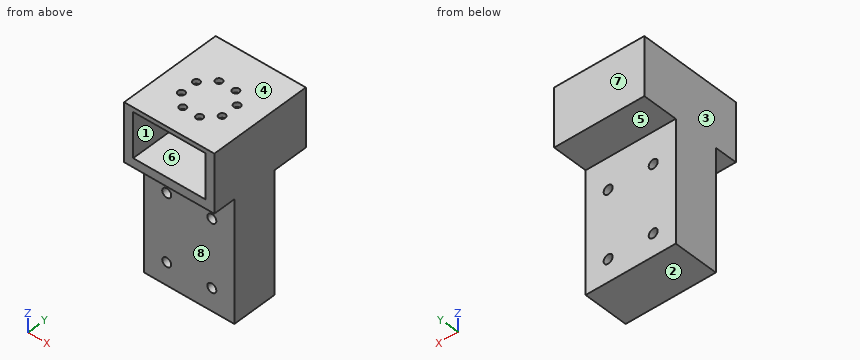
from build123d import *

# Parameters (mm, degrees)
CROQUIS1_W              = 40
CROQUIS1_H              = 40
SALIENTE_EXTRUIR1_DEPTH = 4
CROQUIS2_R              = 1.5
CORTAR_EXTRUIR1_DEPTH   = 4
SALIENTE_EXTRUIR2_DEPTH = 20
CROQUIS4_W              = 40
CROQUIS4_H              = 40
SALIENTE_EXTRUIR3_DEPTH = 4
CROQUIS6_W              = 40
CROQUIS6_H              = 40
CORTAR_EXTRUIR3_DEPTH   = 2
CROQUIS7_W              = 40
CROQUIS7_H              = 20
SALIENTE_EXTRUIR4_DEPTH = 80
CROQUIS8_R              = 2
CORTAR_EXTRUIR4_DEPTH   = 31
CROQUIS9_R              = 2
CORTAR_EXTRUIR5_DEPTH   = 31
CROQUIS11_W             = 40
CROQUIS11_H             = 20
CORTAR_EXTRUIR6_DEPTH   = 26
CROQUIS13_W             = 40
CROQUIS13_H             = 26
SALIENTE_EXTRUIR5_DEPTH = 5.7


with BuildPart() as part:
    # Croquis1 → Saliente-Extruir1 (new body)
    with BuildSketch(Plane.XY):
        Rectangle(CROQUIS1_W, CROQUIS1_H)
    extrude(amount=SALIENTE_EXTRUIR1_DEPTH)

    # Croquis2 → Cortar-Extruir1 (cut)
    with BuildSketch(Plane.XY.offset(4)):
        with Locations((-9.034617948, -3.742261285)):
            Circle(CROQUIS2_R)
        with Locations((-9.034617948, 3.742261285)):
            Circle(CROQUIS2_R)
        with Locations((-3.742261285, 9.034617948)):
            Circle(CROQUIS2_R)
        with Locations((3.742261285, 9.034617948)):
            Circle(CROQUIS2_R)
        with Locations((9.034617948, 3.742261285)):
            Circle(CROQUIS2_R)
        with Locations((9.034617948, -3.742261285)):
            Circle(CROQUIS2_R)
        with Locations((3.742261285, -9.034617948)):
            Circle(CROQUIS2_R)
        with Locations((-3.742261285, -9.034617948)):
            Circle(CROQUIS2_R)
    extrude(amount=-CORTAR_EXTRUIR1_DEPTH, mode=Mode.SUBTRACT)

    # Croquis3 → Saliente-Extruir2 (add)
    with BuildSketch(Plane(origin=(0, 0, 0), x_dir=(-1, 0, 0), z_dir=(0, 0, -1))):
        Polygon((-16, -20), (-16, -16), (-16, 16), (16, 16), (16, -16), (16, -20), (20, -20), (20, 20), (-20, 20), (-20, -20), align=None)
    extrude(amount=SALIENTE_EXTRUIR2_DEPTH)

    # Croquis4 → Saliente-Extruir3 (add)
    with BuildSketch(Plane(origin=(0, 0, -20), x_dir=(-1, 0, 0), z_dir=(0, 0, -1))):
        Rectangle(CROQUIS4_W, CROQUIS4_H)
    extrude(amount=SALIENTE_EXTRUIR3_DEPTH)

    # Croquis6 → Cortar-Extruir3 (cut)
    with BuildSketch(Plane.XY.offset(4)):
        Rectangle(CROQUIS6_W, CROQUIS6_H)
    extrude(amount=-CORTAR_EXTRUIR3_DEPTH, mode=Mode.SUBTRACT)

    # Croquis7 → Saliente-Extruir4 (add)
    with BuildSketch(Plane(origin=(0, 0, -24), x_dir=(-1, 0, 0), z_dir=(0, 0, -1))):
        Rectangle(CROQUIS7_W, CROQUIS7_H)
    extrude(amount=SALIENTE_EXTRUIR4_DEPTH)

    # Croquis8 → Cortar-Extruir4 (cut, through all)
    with BuildSketch(Plane(origin=(0, 10, 0), x_dir=(1, 0, 0), z_dir=(0, 1, 0))):
        with Locations((-10, 38)):
            Circle(CROQUIS8_R)
        with Locations((10, 38)):
            Circle(CROQUIS8_R)
    extrude(amount=-CORTAR_EXTRUIR4_DEPTH, mode=Mode.SUBTRACT)

    # Croquis9 → Cortar-Extruir5 (cut, through all)
    with BuildSketch(Plane(origin=(0, 10, 0), x_dir=(1, 0, 0), z_dir=(0, 1, 0))):
        with Locations((10, 68)):
            Circle(CROQUIS9_R)
        with Locations((-10, 68)):
            Circle(CROQUIS9_R)
    extrude(amount=-CORTAR_EXTRUIR5_DEPTH, mode=Mode.SUBTRACT)

    # Croquis11 → Cortar-Extruir6 (cut)
    with BuildSketch(Plane(origin=(0, 0, -104), x_dir=(-1, 0, 0), z_dir=(0, 0, -1))):
        Rectangle(CROQUIS11_W, CROQUIS11_H)
    extrude(amount=-CORTAR_EXTRUIR6_DEPTH, mode=Mode.SUBTRACT)

    # Croquis13 → Saliente-Extruir5 (add)
    with BuildSketch(Plane(origin=(0, 20, 0), x_dir=(1, 0, 0), z_dir=(0, 1, 0))):
        with Locations((0, 11)):
            Rectangle(CROQUIS13_W, CROQUIS13_H)
    extrude(amount=SALIENTE_EXTRUIR5_DEPTH)


solid = part.part
Geometry check sheet. Reference: the model listing, model coordinates, mm. Face numbers are marked on the shaded views. A direction names the side the tool comes from. Coordinates: 2 decimals unless noted, no trailing zeros. Loops run counter-clockwise (first coordinate to the right, second up) from the corner with the lowest first, then second, coordinate; pieces in that order, holes last. Notation, with made-up numbers: (-26, -39) - (10, -39) arc R20 ccw to (10, -9) - close; hole circle Ø5 at (78, 39.25). An arc over 180 degrees is marked (long way). Use one line per item in the form item = value. Start each with the question number.
Item 1: Thickness scan on probe 1 along Z at (x, y) = (10, 5); probe 2 along X at (y, z) = (4.75, -38); probe 3 along Z at (x, y) = (-5, -7.5). Record the ranges inside material, lowest first.
Item 2: Section check A-A, the plane z = -68. Enter the section's corners in (x, y).
Item 3: Mould release check, pull along Z, two halves, no side actions. Record for the marked faces 1, 2, 3 and 4: +Z half, -Z half, draft (parallel to the pull), parting line (faces both ways), or undercut.
Item 4: Section check B-B, the plane x = 17. Enter the section's corners in (y, z).
Item 5: Tool access check on the marked faces 5, 6, 7 and 8. Record the directions out of +Z, -Z, +X, -X, +Y, -Y that give a thin tool (end or side, any length) a straight path to the whole face; none if there is none.
Item 6: Section check C-C, the plane z = -6. Enter the section's corners in (x, y).
Item 7: Gauge pin test, flat ends, axial feed: pin 1 (4.5 mm diameter, centred on x = 10, z = -68, fed in from -Y); pin 2 (6 mm diameter, centred on x = 0.5, z = -39.5, fed in from +Y). Record the tip position at first contact, or that the pin passes through.
Computed:
q1.probe_1 = -78 to -70, -66 to -40, -36 to -20, 0 to 2
q1.probe_2 = -20 to -12, -8 to 8, 12 to 20
q1.probe_3 = -78 to -20, 0 to 2
q2.outline = (-20, -10) - (-12, -10) - (-12, 10) - (-20, 10) - close; (-8, -10) - (8, -10) - (8, 10) - (-8, 10) - close; (12, -10) - (20, -10) - (20, 10) - (12, 10) - close
q3.face_1 = undercut
q3.face_2 = -Z half
q3.face_3 = draft
q3.face_4 = +Z half
q4.outline = (-20, -24) - (-10, -24) - (-10, -78) - (10, -78) - (10, -24) - (25.7, -24) - (25.7, 2) - (-20, 2) - close
q5.face_5 = -Z, +X, -X, +Y
q5.face_6 = -Y
q5.face_7 = +Z, -Z, +X, -X, +Y
q5.face_8 = -Z, +X, -X, -Y
q6.outline = (-20, -20) - (-16, -20) - (-16, 16) - (16, 16) - (16, -20) - (20, -20) - (20, 25.7) - (-20, 25.7) - close
q7.pin_1 = -10
q7.pin_2 = 10
